from build123d import *

# Parameters (mm, degrees)
F2_DEPTH = 200


with BuildPart() as f2:
    # F0 (on Front) → F2 (new body)
    with BuildSketch(Plane.XZ):
        with BuildLine():
            Line((-10, 0), (0, 0))
            Line((0, 0), (10, 0))
            Line((10, 0), (10, 4))
            ThreePointArc((10, 4), (8.2820023216, 6.4560436706), (9.8669164293, 9))
            Line((9.8669164293, 9), (9.8669164293, 10))
            Line((9.8669164293, 10), (0, 10))
            Line((0, 10), (-9.8669164293, 10))
            Line((-9.8669164293, 10), (-9.8669164293, 9))
            ThreePointArc((-9.8669164293, 9), (-8.2820023216, 6.4560436706), (-10, 4))
            Line((-10, 4), (-10, 0))
        make_face()
    extrude(amount=F2_DEPTH)


solid = f2.part
Read the model definition and answer for the solid it produces. Units are mm, in the model's axes. Coordinates: 2 decimals unless noted, no trailing zeros. Write each loop counter-clockwise with the first axis right and the second up, starting at its lowest first coordinate (ties: lowest second). Pieces come first, ordered by that corner, then holes. Notation, with made-up numbers: M 2.5,43 L 28.5,43 A29 cw 28.5,78 Z; hole C 48.5,67.25 d2. An arc over 180 degrees is marked long. Use a Markdown table: item, result.
Q1. This flat-tipped pin is pushed along its axis until it touches: pin 1 Ø0.8 at (y, z) = (-64.5, 9.5) entering from +X. Where does it stop, or does it pass through?
Answer block:
| item | result |
|---|---|
| pin 1 | stops at x = 9.87 |
Q2. Straight lines are drawn through the part: L1, parallel to X at y = -117, z = 6.75; L2, parallel to X at y = -106.5, z = 9.25. For each, find the intervals that lie inside material, in ascending order. Write a range as [from, to].
Answer block:
| item | result |
|---|---|
| L1 | x = [-8.29, 8.29] |
| L2 | x = [-9.87, 9.87] |
Q3. The part is cut by section A-A, the plane y = -19. Write down the section's boundary in (x, z), then the cut area to 3 significant figures.
Answer block:
| item | result |
|---|---|
| outline | M -10,0 L 10,0 L 10,4 A2.72 cw 9.87,9 L 9.87,10 L -9.87,10 L -9.87,9 A2.72 cw -10,4 Z |
| area | 187 mm2 |
Q4. Determine the mould class of faces 1 (the face through (0, -99, 0)), 2 (the face through (0, -99, 10)), 3 (the face through (8.284, -98.6, 6.412)) for opening direction Z: released by +Z, released by -Z, zero draft, split by the parting line, or undercut.
Answer block:
| item | result |
|---|---|
| face 1 | released by -Z |
| face 2 | released by +Z |
| face 3 | undercut |
